Autodesk Inventor part; units mm, degrees
ref_plane "YZ Plane" through (0, 0, 0) normal (1, 0, 0) x (0, 1, 0)
ref_plane "XZ Plane" through (0, 0, 0) normal (0, 1, 0) x (-1, 0, 0)
ref_plane "XY Plane" through (0, 0, 0) normal (0, 0, 1) x (1, 0, 0)
sketch "Sketch1" plane through (0, 0, 0) normal (0, 0, 1) x (1, 0, 0)
  line L0 (-25, -30) -> (25, -30)
  line L1 (52, -3) -> (52, 3)
  line L2 (25, 30) -> (-25, 30)
  line L3 (-52, 3) -> (-52, -3)
  line L4 (-52, -30) -> (52, 30) construction
  line L5 (52, -30) -> (-52, 30) construction
  arc A0 (-25, 30) -> (-52, 3) centre (-25, 3) ccw
  arc A1 (52, 3) -> (25, 30) centre (25, 3) ccw
  arc A2 (25, -30) -> (52, -3) centre (25, -3) ccw
  arc A3 (-52, -3) -> (-25, -30) centre (-25, -3) ccw
  line L6 (-51.1, 3) -> (-51.1, -3)
  arc A4 (-51.1, -3) -> (-25, -29.1) centre (-25, -3) ccw
  line L7 (-25, -29.1) -> (25, -29.1)
  arc A5 (25, -29.1) -> (51.1, -3) centre (25, -3) ccw
  line L8 (51.1, -3) -> (51.1, 3)
  arc A6 (51.1, 3) -> (25, 29.1) centre (25, 3) ccw
  line L9 (25, 29.1) -> (-25, 29.1)
  arc A7 (-25, 29.1) -> (-51.1, 3) centre (-25, 3) ccw
  line L10 (-25, 28) -> (25, 28)
  arc A8 (50, 3) -> (25, 28) centre (25, 3) ccw
  line L11 (50, 3) -> (50, -7)
  line L12 (-50, -7) -> (-50, 3)
  arc A9 (-25, 28) -> (-50, 3) centre (-25, 3) ccw
  line L13 (-50, -7) -> (50, -7)
  line L14 (-34.5, -8.5) -> (-25.5, -8.5)
  line L15 (-25.5, -8.5) -> (-25.5, -17.5)
  line L16 (-25.5, -17.5) -> (-34.5, -17.5)
  line L17 (-34.5, -17.5) -> (-34.5, -8.5)
  line L18 (-24.5, -8.5) -> (-15.5, -8.5)
  line L19 (-24.5, -17.5) -> (-24.5, -8.5)
  line L20 (-15.5, -8.5) -> (-15.5, -17.5)
  line L21 (-15.5, -17.5) -> (-24.5, -17.5)
  line L22 (-14.5, -8.5) -> (-5.5, -8.5)
  line L23 (-14.5, -17.5) -> (-14.5, -8.5)
  line L24 (-5.5, -8.5) -> (-5.5, -17.5)
  line L25 (-5.5, -17.5) -> (-14.5, -17.5)
  line L26 (-4.5, -8.5) -> (4.5, -8.5)
  line L27 (-4.5, -17.5) -> (-4.5, -8.5)
  line L28 (4.5, -8.5) -> (4.5, -17.5)
  line L29 (4.5, -17.5) -> (-4.5, -17.5)
  line L30 (5.5, -8.5) -> (14.5, -8.5)
  line L31 (5.5, -17.5) -> (5.5, -8.5)
  line L32 (14.5, -8.5) -> (14.5, -17.5)
  line L33 (14.5, -17.5) -> (5.5, -17.5)
  line L34 (15.5, -8.5) -> (24.5, -8.5)
  line L35 (15.5, -17.5) -> (15.5, -8.5)
  line L36 (24.5, -8.5) -> (24.5, -17.5)
  line L37 (24.5, -17.5) -> (15.5, -17.5)
  line L38 (25.5, -8.5) -> (34.5, -8.5)
  line L39 (25.5, -17.5) -> (25.5, -8.5)
  line L40 (34.5, -8.5) -> (34.5, -17.5)
  line L41 (34.5, -17.5) -> (25.5, -17.5)
  line L42 (-31.25, -22.5) -> (31.25, -22.5) construction
  line L43 (-31.25, -26) -> (31.25, -26)
  line L44 (31.25, -19) -> (-31.25, -19)
  arc A10 (-31.25, -19) -> (-31.25, -26) centre (-31.25, -22.5) ccw
  arc A11 (31.25, -26) -> (31.25, -19) centre (31.25, -22.5) ccw
  point P0 (0, 0)
  point P1 (0, -22.5)
  point P2 (0, 0)
  point P3 (0, -8.5)
  point P4 (4.5, -13)
  point P5 (0, 0)
  dimension "d0" = 104
  dimension "d1" = 60
  dimension "d2" = 27
  dimension "d3" = 58.2
  dimension "d4" = 2
  dimension "d5" = 23
  dimension "d6" = 9
  dimension "d9" = 10
  dimension "d16" = 62.5
  dimension "d17" = 7
  dimension "d24" = 13
  dimension "d25" = 22.5
extrude "Extrusion1" add sketch "Sketch1" against normal blind 2.1 contours A3 L3 A0 L2 A1 L1 A2 L0
extrude "Extrusion2" add sketch "Sketch1" along normal blind 0.8 contours A3 L3 A0 L2 A1 L1 A2 L0 | A7 L9 A6 L8 A5 L7 A4 L6
sketch "Sketch2" plane through (0, 0, -2.1) normal (0, 0, -1) x (-1, 0, 0)
  arc A0 (25, -29.1) -> (51.1, -3) centre (25, -3) ccw
  line L0 (25, -29.1) -> (-25, -29.1)
  arc A1 (-51.1, -3) -> (-25, -29.1) centre (-25, -3) ccw
  line L1 (-51.1, -3) -> (-51.1, 3)
  arc A2 (-25, 29.1) -> (-51.1, 3) centre (-25, 3) ccw
  line L2 (-25, 29.1) -> (25, 29.1)
  arc A3 (51.1, 3) -> (25, 29.1) centre (25, 3) ccw
  line L3 (51.1, 3) -> (51.1, -3)
  line L4 (25, 30) -> (-25, 30)
  arc A4 (-25, 30) -> (-52, 3) centre (-25, 3) ccw
  line L5 (-52, 3) -> (-52, -3)
  arc A5 (-52, -3) -> (-25, -30) centre (-25, -3) ccw
  line L6 (-25, -30) -> (25, -30)
  arc A6 (25, -30) -> (52, -3) centre (25, -3) ccw
  line L7 (52, -3) -> (52, 3)
  arc A7 (52, 3) -> (25, 30) centre (25, 3) ccw
  line L8 (51.1, 3) -> (51.1, -3)
  line L9 (51.1, -1.7321) -> (50.1, 0)
  line L10 (50.1, 0) -> (51.1, 1.7321)
  point P0 (0, 0)
  point P1 (51.1, 0)
  dimension "d26" = 1
  dimension "d27" = 120
extrude "Extrusion3" add sketch "Sketch2" against normal up to surface (2.1 mm away) contours L9 L10 L3
mirror "Mirror1" about plane through (0, 0, 0) normal (1, 0, 0) of "Extrusion3"
properties part number "Game_ColoniesV2"
Design review of the part built by this model. Coordinates are the model's own, in mm. A direction names the side the tool comes from. Coordinates: 2 decimals unless noted, no trailing zeros. Order: outer loops, then holes, each group sorted by start corner. A loop starts at its lowest first (then second) coordinate and runs counter-clockwise, first axis right, second up. Notation, with made-up numbers: (-36, 40) - (10, 40) arc R16 ccw to (10, 52) - close; hole circle Ø10 at (13, -4.5). An arc over 180 degrees is marked (long way). Answer in a Markdown table with one row per item.
(1) Consider section A-A on x = -13. State the section outline as (y, z) points, plus the area to 3 significant figures.
Checked values:
| item | result |
|---|---|
| outline | (-30, -2.1) - (-29.1, -2.1) - (-29.1, 0) - (-26, 0) - (-26, 0.8) - (-30, 0.8) - close; (-19, 0) - (-17.5, 0) - (-17.5, 0.8) - (-19, 0.8) - close; (-8.5, 0) - (-7, 0) - (-7, 0.8) - (-8.5, 0.8) - close; (28, 0) - (29.1, 0) - (29.1, -2.1) - (30, -2.1) - (30, 0.8) - (28, 0.8) - close |
| area | 11.0 mm^2 |
(2) Consider section D-D on x = 39. State the section outline as (y, z) points.
Checked values:
| item | result |
|---|---|
| outline | (-26.09, -2.1) - (-25.03, -2.1) - (-25.03, 0) - (-7, 0) - (-7, 0.8) - (-26.09, 0.8) - close; (23.71, 0) - (25.03, 0) - (25.03, -2.1) - (26.09, -2.1) - (26.09, 0.8) - (23.71, 0.8) - close |
(3) Consider section B-B on z = -0.7. State the section outline as (x, y) points.
Checked values:
| item | result |
|---|---|
| outline | (-52, -3) arc R27 ccw to (-25, -30) - (25, -30) arc R27 ccw to (52, -3) - (52, 3) arc R27 ccw to (25, 30) - (-25, 30) arc R27 ccw to (-52, 3) - close; hole (-51.1, -3) arc R26.1 ccw to (-25, -29.1) - (25, -29.1) arc R26.1 ccw to (51.1, -3) - (51.1, -1.73) - (50.1, 0) - (51.1, 1.73) - (51.1, 3) arc R26.1 ccw to (25, 29.1) - (-25, 29.1) arc R26.1 ccw to (-51.1, 3) - (-51.1, 1.73) - (-50.1, 0) - (-51.1, -1.73) - close |
(4) For faces 4 (the cylindrical face through (43.25, -21.66, -1.04)), 5 (the flat face through (-52, 0, -1)), 6 (the cylindrical face through (42.482, 20.871, 0.394)), list the 3-axis set-ups (+Z, -Z, +X, -X, +Y, -Y) from which the entire face can be reached by the end or side of a thin tool; tool diameter is ignored.
Checked values:
| item | result |
|---|---|
| face 4 | -Z |
| face 5 | +Z, -Z, -X, +Y, -Y |
| face 6 | +Z, -Z |
(5) Consider section C-C on y = 15. State the section outline as (x, z) points.
Checked values:
| item | result |
|---|---|
| outline | (-49.19, -2.1) - (-48.18, -2.1) - (-48.18, 0) - (-46.93, 0) - (-46.93, 0.8) - (-49.19, 0.8) - close; (46.93, 0) - (48.18, 0) - (48.18, -2.1) - (49.19, -2.1) - (49.19, 0.8) - (46.93, 0.8) - close |
(6) Clearance check with flat-ended pins moving along their axes: pin 1 (0.9 mm diameter, centred on x = 28, z = 0.5, fed in from +Y); pin 2 (1 mm diameter, centred on y = -9.5, z = -1, fed in from +X); pin 3 (10 mm diameter, centred on x = 14, y = -22.5, fed in from -Z). State where each tip first meets the part, or that it passes through.
Checked values:
| item | result |
|---|---|
| pin 1 | y = 29.88 |
| pin 2 | x = 51.32 |
| pin 3 | z = 0 |
(7) The part is to be moulded in two halves that separate along X. For faces 1 (the cylindrical face through (-43.66, -21.25, -1.04)), 2 (the flat face through (52, 0, -1)), 3 (the flat face through (-31, 29, -2.1)), say which applies: released by +X, released by -X, zero draft, split by the parting line, or undercut.
Checked values:
| item | result |
|---|---|
| face 1 | undercut |
| face 2 | released by +X |
| face 3 | zero draft |
(8) Wall thickness on line 1 along Y through (x, z) = (-11.5, 0.55); line 2 along Y through (x, z) = (-5, 0.1); line 3 along X through (y, z) = (-2, -0.5): over which ranges is each line inside the solid? List them lowest first. Write a range as from..to.
Checked values:
| item | result |
|---|---|
| line 1 | -30..-26, -19..-17.5, -8.5..-7, 28..30 |
| line 2 | -30..-26, -19..-7, 28..30 |
| line 3 | -52..-51.1, 51.1..52 |
